Verification items for the finished model (mm, model axes). Face numbers are marked on the shaded views. A direction names the side the tool comes from. Give positions to 0.01 mm unless a question says otherwise; leave off trailing zeros. Loops run counter-clockwise (first coordinate to the right, second up) from the corner with the lowest first, then second, coordinate; pieces in that order, holes last. Notation, with made-up numbers: M -5.75,32.25 L 1.25,32.25 A21 cw 1.25,60.25 Z; hole C 29.5,6.5 d7. An arc over 180 degrees is marked long. Put each result on its own line as item: value. Start each with the question number.
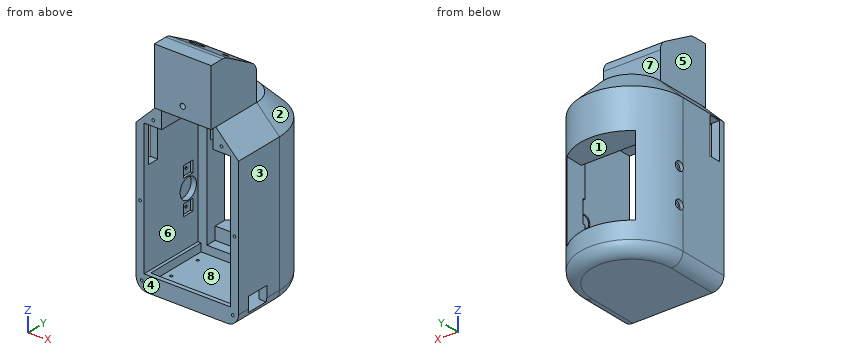
from build123d import *

# Parameters (mm, degrees)
SCHIZZO1_W                             = 90
SCHIZZO1_H                             = 150
ESTRUSIONE_ESTRUSIONE1_DEPTH           = 90
SCHIZZO4_W                             = 60
SCHIZZO4_H                             = 70
TAGLIO_ESTRUSIONE2_DEPTH               = 90
RACCORDO5_R                            = 45
RACCORDO6_R                            = 45
SMUSSO2_SIZE                           = 20
SCHIZZO7_W                             = 50
SCHIZZO7_H                             = 44.753189799
ESTRUSIONE_ESTRUSIONE2_DEPTH           = 50
SMUSSO3_SIZE                           = 20
SMUSSO3_SIZE2                          = 34.641016151
RACCORDO7_R                            = 10
RACCORDO8_R                            = 10
SCHIZZO9_W                             = 50
SCHIZZO9_H                             = 50
ESTRUSIONE_ESTRUSIONE3_DEPTH           = 5
RACCORDO9_R                            = 10
SCHIZZO13_W                            = 45
SCHIZZO13_H                            = 38.415996799
TAGLIO_ESTRUSIONE3_DEPTH               = 79.978264331
SCHIZZO14_W                            = 117.844501366
SCHIZZO14_H                            = 59.041021869
TAGLIO_ESTRUSIONE4_DEPTH               = 8
SCHIZZO18_R                            = 5
TAGLIO_ESTRUSIONE5_DEPTH               = 9
SCHIZZO16_W                            = 4
SCHIZZO16_H                            = 20
TAGLIO_ESTRUSIONE7_DEPTH               = 2
SCHIZZO23_W                            = 76
SCHIZZO23_H                            = 117.844501366
TAGLIO_ESTRUSIONE8_DEPTH               = 38
FORO_PER_VITE_M2_2_D                   = 2.4
FORO_PER_VITE_M2_2_DEPTH               = 4
FORO_PER_VITE_M4_1_D                   = 4.5
FORO_PER_VITE_M4_1_DEPTH               = 10
SCHIZZO29_W                            = 60
SCHIZZO29_H                            = 11.209863528
TAGLIO_ESTRUSIONE9_DEPTH               = 30
SCHIZZO30_W                            = 70
SCHIZZO30_H                            = 52
TAGLIO_ESTRUSIONE10_DEPTH              = 7
FORO_PER_VITE_M2_3_D                   = 2.4
FORO_PER_VITE_M2_3_DEPTH               = 4
FORO_PER_VITE_M2_3_TIP                 = 0.721032743
SCHIZZO33_W                            = 13
SCHIZZO33_H                            = 20
TAGLIO_ESTRUSIONE11_DEPTH              = 36
SCHIZZO36_W                            = 46.07976418
SCHIZZO36_H                            = 28.262497783
TAGLIO_ESTRUSIONE12_DEPTH              = 28
ESTRUSIONE_ESTRUSIONE4_REACH           = 170.388
SCHIZZO38_R                            = 6
SCHIZZO38_R_2                          = 2.5
TAGLIO_ESTRUSIONE13_DEPTH              = 28
SCHIZZO39_R                            = 9
SCHIZZO39_W                            = 10
SCHIZZO39_H                            = 10
TAGLIO_ESTRUSIONE14_DEPTH              = 2
SCHIZZO40_W                            = 32
SCHIZZO40_H                            = 10
TAGLIO_ESTRUSIONE15_DEPTH              = 10
SCHIZZO42_R                            = 4
TAGLIO_ESTRUSIONE16_DEPTH              = 3
FORO_SVASATO_PER_VITE_M2_3_D           = 2.4
FORO_SVASATO_PER_VITE_M2_3_DEPTH       = 6
FORO_SVASATO_PER_VITE_M2_3_CSINK_D     = 4.4
FORO_SVASATO_PER_VITE_M2_3_CSINK_ANGLE = 90
FORO_SVASATO_PER_VITE_M2_3_TIP         = 0.721032743
TAGLIO_ESTRUSIONE18_DEPTH              = 7
SCHIZZO53_R                            = 9
TAGLIO_ESTRUSIONE19_DEPTH              = 2.75
SCHIZZO54_W                            = 60
SCHIZZO54_H                            = 36.634637838
TAGLIO_ESTRUSIONE20_DEPTH              = 24.75


with BuildPart() as part:
    # Schizzo1 → Estrusione-Estrusione1 (new body)
    with BuildSketch(Plane(origin=(0, 0, 0), x_dir=(1, 0, 0), z_dir=(0, 1, 0))):
        Rectangle(SCHIZZO1_W, SCHIZZO1_H)
    extrude(amount=ESTRUSIONE_ESTRUSIONE1_DEPTH)

    # Schizzo4 → Taglio-Estrusione2 (cut)
    with BuildSketch(Plane(origin=(0, 90, 0), x_dir=(1, 0, 0), z_dir=(0, 1, 0))):
        with Locations((0, 15)):
            Rectangle(SCHIZZO4_W, SCHIZZO4_H)
    extrude(amount=-TAGLIO_ESTRUSIONE2_DEPTH, mode=Mode.SUBTRACT)

    # Raccordo5
    # the kernel refuses this fillet: 45 mm, written as the material it takes off along each edge
    with BuildSketch(Plane(origin=(-45, 90, -187.5), x_dir=(0, -1, 0), z_dir=(0, 0, 1))) as raccordo5_piece_1:
        with BuildLine():
            CenterArc((RACCORDO5_R, RACCORDO5_R), RACCORDO5_R, 180, 90)
            Line((0, RACCORDO5_R), (0, 0))
            Line((0, 0), (RACCORDO5_R, 0))
        make_face()
    extrude(amount=375, mode=Mode.SUBTRACT)

    # Raccordo6
    # the kernel refuses this fillet: 45 mm, written as the material it takes off along each edge
    with BuildSketch(Plane(origin=(45, 90, 187.5), x_dir=(0, -1, 0), z_dir=(0, 0, -1))) as raccordo6_piece_1:
        with BuildLine():
            CenterArc((RACCORDO6_R, RACCORDO6_R), RACCORDO6_R, 180, 90)
            Line((0, RACCORDO6_R), (0, 0))
            Line((0, 0), (RACCORDO6_R, 0))
        make_face()
    extrude(amount=375, mode=Mode.SUBTRACT)

    # Smusso2
    smusso2_edges = [part.edges().sort_by_distance(p)[0] for p in [
        (-45, 22.5, 75),
        (0, 90, 75),
        (45, 22.5, 75),
        (0, 90, 75),
    ]]
    chamfer(smusso2_edges, length=SMUSSO2_SIZE)

    # Schizzo7 → Estrusione-Estrusione2 (add)
    with BuildSketch(Plane.XY.offset(75)):
        with Locations((0, 22.3765949)):
            Rectangle(SCHIZZO7_W, SCHIZZO7_H)
    extrude(amount=ESTRUSIONE_ESTRUSIONE2_DEPTH)

    # Smusso3
    smusso3_edges = [part.edges().sort_by_distance(p)[0] for p in [
        (0, 44.753189799, 125),
    ]]
    smusso3_side = [part.faces().sort_by_distance(p)[0] for p in [
        (0, 44.753189799, 100),
    ]]
    chamfer(smusso3_edges, length=SMUSSO3_SIZE, length2=SMUSSO3_SIZE2, reference=smusso3_side[0])

    # Raccordo7
    raccordo7_edges = [part.edges().sort_by_distance(p)[0] for p in [
        (0, 44.753189799, 105),
    ]]
    fillet(raccordo7_edges, radius=RACCORDO7_R)

    # Raccordo8
    raccordo8_edges = [part.edges().sort_by_distance(p)[0] for p in [
        (0, 10.112173648, 125),
    ]]
    fillet(raccordo8_edges, radius=RACCORDO8_R)

    # Schizzo9 → Estrusione-Estrusione3 (add)
    with BuildSketch(Plane.XZ):
        with Locations((0, 100)):
            Rectangle(SCHIZZO9_W, SCHIZZO9_H)
    extrude(amount=ESTRUSIONE_ESTRUSIONE3_DEPTH)

    # Raccordo9
    raccordo9_edges = [part.edges().sort_by_distance(p)[0] for p in [
        (-45, 22.5, -75),
        (0, 90, -75),
        (45, 22.5, -75),
        (0, 90, -75),
    ]]
    fillet(raccordo9_edges, radius=RACCORDO9_R)

    # Schizzo13 → Taglio-Estrusione3 (cut)
    with BuildSketch(Plane(origin=(0, 0, 20), x_dir=(-1, 0, 0), z_dir=(0, 0, -1))):
        with Locations((0, 19.2079984)):
            Rectangle(SCHIZZO13_W, SCHIZZO13_H)
    extrude(amount=-TAGLIO_ESTRUSIONE3_DEPTH, mode=Mode.SUBTRACT)

    # Schizzo14 → Taglio-Estrusione4 (cut)
    with BuildSketch(Plane.ZY.offset(-30)):
        with Locations((-2.287612845, 29.520510935)):
            Rectangle(SCHIZZO14_W, SCHIZZO14_H)
    taglio_estrusione4 = extrude(amount=-TAGLIO_ESTRUSIONE4_DEPTH, mode=Mode.SUBTRACT)

    # Specchia1: Taglio-Estrusione4 across plane
    add(taglio_estrusione4.mirror(Plane(origin=(0, 0, 0), x_dir=(0, 0, 1), z_dir=(1, 0, 0))), mode=Mode.SUBTRACT)

    # Schizzo18 → Taglio-Estrusione5 (cut)
    with BuildSketch(Plane.ZY.offset(-30)):
        with Locations((-15, 48.541019662)):
            Circle(SCHIZZO18_R)
    extrude(amount=-TAGLIO_ESTRUSIONE5_DEPTH, mode=Mode.SUBTRACT)

    # Schizzo16 → Taglio-Estrusione7 (cut)
    with BuildSketch(Plane.XZ.offset(-59.041021869)):
        with Locations((32, -15)):
            Rectangle(SCHIZZO16_W, SCHIZZO16_H)
    extrude(amount=-TAGLIO_ESTRUSIONE7_DEPTH, mode=Mode.SUBTRACT)

    # Schizzo23 → Taglio-Estrusione8 (cut)
    with BuildSketch(Plane.XZ):
        with Locations((0, -2.287612845)):
            Rectangle(SCHIZZO23_W, SCHIZZO23_H)
    extrude(amount=-TAGLIO_ESTRUSIONE8_DEPTH, mode=Mode.SUBTRACT)

    # Foro per Vite M2-2
    with Locations(Plane(origin=(0, 0, 0), x_dir=(-1, 0, 0), z_dir=(0, -1, 0))):
        with Locations((40, 67), (30, -61.514718626), (-30, -61.514718626), (-40, 67), (-41.5, 5), (41.5, 5)):
            Hole(FORO_PER_VITE_M2_2_D / 2, depth=FORO_PER_VITE_M2_2_DEPTH)

    # Foro per Vite M4-1
    with Locations(Plane(origin=(0, -5, 84.779580177), x_dir=(0, 0, -1), z_dir=(0, -1, 0))):
        with Locations((0, 0)):
            Hole(FORO_PER_VITE_M4_1_D / 2, depth=FORO_PER_VITE_M4_1_DEPTH)

    # Schizzo29 → Taglio-Estrusione9 (cut)
    with BuildSketch(Plane.XZ.offset(-38)):
        with Locations((0, -55.604931764)):
            Rectangle(SCHIZZO29_W, SCHIZZO29_H)
    extrude(amount=-TAGLIO_ESTRUSIONE9_DEPTH, mode=Mode.SUBTRACT)

    # Schizzo30 → Taglio-Estrusione10 (cut)
    with BuildSketch(Plane.XY.offset(-61.209863528)):
        with Locations((3, 29.778767455)):
            Rectangle(SCHIZZO30_W, SCHIZZO30_H)
    extrude(amount=-TAGLIO_ESTRUSIONE10_DEPTH, mode=Mode.SUBTRACT)

    # Foro per Vite M2-3
    with Locations(Plane.XY.offset(-68.209863528)):
        with Locations((-29.5, 48.278767455), (-29.5, 19.278767455), (22.5, 6.278767455), (22.5, 53.278767455)):
            Hole(FORO_PER_VITE_M2_3_D / 2, depth=FORO_PER_VITE_M2_3_DEPTH)
            with Locations((0, 0, -(FORO_PER_VITE_M2_3_DEPTH + FORO_PER_VITE_M2_3_TIP / 2))):  # 118° drill point
                Cone(0, FORO_PER_VITE_M2_3_D / 2, FORO_PER_VITE_M2_3_TIP, mode=Mode.SUBTRACT)

    # Schizzo33 → Taglio-Estrusione11 (cut)
    with BuildSketch(Plane.ZY.offset(-38)):
        with Locations((-61.709863528, 21)):
            Rectangle(SCHIZZO33_W, SCHIZZO33_H)
    extrude(amount=-TAGLIO_ESTRUSIONE11_DEPTH, mode=Mode.SUBTRACT)

    # Schizzo36 → Taglio-Estrusione12 (cut)
    with BuildSketch(Plane(origin=(0, 56.654631148, 98.128699633), x_dir=(1, 0, 0), z_dir=(0, 0.5000000000000012, 0.8660254037844378))):
        with Locations((0, -35.289606117)):
            Rectangle(SCHIZZO36_W, SCHIZZO36_H)
    extrude(amount=-TAGLIO_ESTRUSIONE12_DEPTH, mode=Mode.SUBTRACT)

    # Schizzo37 → Estrusione-Estrusione4 (add, up to next)
    with BuildSketch(Plane.ZY.offset(-23.03988209), mode=Mode.PRIVATE) as estrusione_estrusione4_sk1:
        Polygon((122.839127138, 13.854915234), (108.707878246, 38.330956288), (106.809101084, 37.234696782), (120.940349975, 12.758655728), align=None)
    estrusione_estrusione4_tool1 = extrude(estrusione_estrusione4_sk1.sketch, amount=ESTRUSIONE_ESTRUSIONE4_REACH, mode=Mode.PRIVATE) - part.part
    add(estrusione_estrusione4_tool1.solids().sort_by_distance((23.039882, 25.544806, 114.824114))[0])

    # Schizzo38 → Taglio-Estrusione13 (cut)
    with BuildSketch(Plane(origin=(0, 56.654631148, 98.128699633), x_dir=(1, 0, 0), z_dir=(0, 0.5000000000000013, 0.8660254037844379))):
        with Locations(Location((-12.5, -35.289606117, 0), (0, 0, 270))):
            Circle(SCHIZZO38_R)
        with Locations(Location((12.5, -35.289606117, 0), (0, 0, 270))):
            Circle(SCHIZZO38_R_2)
    extrude(amount=-TAGLIO_ESTRUSIONE13_DEPTH, mode=Mode.SUBTRACT)

    # Schizzo39 → Taglio-Estrusione14 (cut)
    with BuildSketch(Plane(origin=(-38, 0, 0), x_dir=(0, 0, -1), z_dir=(1, 0, 0))):
        with Locations(Location((15, 48.541019662, 0), (0, 0, 90))):
            Circle(SCHIZZO39_R)
        with Locations((0, 48.541019662)):
            Rectangle(SCHIZZO39_W, SCHIZZO39_H)
        with Locations((30, 48.541019662)):
            Rectangle(SCHIZZO39_W, SCHIZZO39_H)
    extrude(amount=-TAGLIO_ESTRUSIONE14_DEPTH, mode=Mode.SUBTRACT)

    # Schizzo40 → Taglio-Estrusione15 (cut)
    with BuildSketch(Plane.ZY.offset(45)):
        with Locations((38, 10)):
            Rectangle(SCHIZZO40_W, SCHIZZO40_H)
    extrude(amount=-TAGLIO_ESTRUSIONE15_DEPTH, mode=Mode.SUBTRACT)

    # Schizzo42 → Taglio-Estrusione16 (cut)
    with BuildSketch(Plane.ZY.offset(45)):
        with Locations((-30, 48.541019662)):
            Circle(SCHIZZO42_R)
        with Locations((0, 48.541019662)):
            Circle(SCHIZZO42_R)
    extrude(amount=-TAGLIO_ESTRUSIONE16_DEPTH, mode=Mode.SUBTRACT)

    # Foro svasato per Vite M2-3
    with Locations(Plane.ZY.offset(42)):
        with Locations((-30, 48.541019662), (0, 48.541019662)):
            CounterSinkHole(FORO_SVASATO_PER_VITE_M2_3_D / 2, FORO_SVASATO_PER_VITE_M2_3_CSINK_D / 2, depth=FORO_SVASATO_PER_VITE_M2_3_DEPTH, counter_sink_angle=FORO_SVASATO_PER_VITE_M2_3_CSINK_ANGLE)
            with Locations((0, 0, -(FORO_SVASATO_PER_VITE_M2_3_DEPTH + FORO_SVASATO_PER_VITE_M2_3_TIP / 2))):  # 118° drill point
                Cone(0, FORO_SVASATO_PER_VITE_M2_3_D / 2, FORO_SVASATO_PER_VITE_M2_3_TIP, mode=Mode.SUBTRACT)

    # Schizzo50 → Taglio-Estrusione18 (cut)
    with BuildSketch(Plane.XY.offset(-61.209863528)):
        Polygon((38, 59.041021869), (38, 55.778767455), (-32, 55.778767455), (-32, 3.778767455), (-35.181345979, 3.778767455), (-35.181345979, 59.041021869), align=None)
    extrude(amount=-TAGLIO_ESTRUSIONE18_DEPTH, mode=Mode.SUBTRACT)

    # Schizzo53 → Taglio-Estrusione19 (cut)
    with BuildSketch(Plane(origin=(-40, 0, 0), x_dir=(0, 0, -1), z_dir=(1, 0, 0))):
        with Locations(Location((15, 48.541019662, 0), (0, 0, 90))):
            Circle(SCHIZZO53_R)
    extrude(amount=-TAGLIO_ESTRUSIONE19_DEPTH, mode=Mode.SUBTRACT)

    # Schizzo54 → Taglio-Estrusione20 (cut)
    with BuildSketch(Plane.XZ.offset(-38)):
        with Locations((0, 38.317318919)):
            Rectangle(SCHIZZO54_W, SCHIZZO54_H)
    extrude(amount=-TAGLIO_ESTRUSIONE20_DEPTH, mode=Mode.SUBTRACT)


solid = part.part
Q1. Cross-section at D-D, the plane z = 94. Record the boundary of the cut face in (x, y), then the cut area to 3 significant figures.
Q2. Cross-section at A-A, the plane z = 11. Record the boundary of the cut face in (x, y).
Q3. Release check for a two-part mould opening along Z. For the marked faces 1, 2 and 3 record: pulls with the +Z half, pulls with the -Z half, needs draft (parallel to the pull), parting line crosses it, or undercut.
Q4. Cross-section at B-B, the plane x = 0. State how many separate pieces and enclosed holes the cut face has, then the cut area to 3 significant figures.
Q5. Cross-section at C-C, the plane z = 45.5. Record the boundary of the cut face in (x, y).
Q6. Scan lines: L1, parallel to X at y = 27, z = -19; L2, parallel to Y at x = -9.5, z = 83.5; L3, parallel to Z at x = -11, y = 34. Record each from-to range of solid material in increasing order.
Q7. Set-up check for the marked faces 4, 5, 6, 7 and 8: record each of +Z, -Z, +X, -X, +Y, -Y from which the full face is reachable in a straight line by a thin tool's end or side.
Q8. Go/stop test with flat-tipped pins: pin 1 (3 mm diameter, centred on x = -27.5, z = -17.5, fed in from -Y) (1 decimal); pin 2 (2.5 mm diameter, centred on y = 48, z = -30.5, fed in from -X); pin 3 (0.9 mm diameter, centred on x = 5, z = 99.5, fed in from +Y); pin 4 (5.5 mm diameter, centred on x = -40.5, y = 9, fed in from +Z). Record where each tip stops, or that it passes through.
Ans:
1. outline: M -25,-5 L 25,-5 L 25,44.75 L -25,44.75 Z; hole M -23.04,7.81 L -22.5,7.81 L -22.5,0 L 22.5,0 L 22.5,7.81 L 23.04,7.81 L 23.04,29.84 L 22.5,29.84 L 22.5,38.42 L -22.5,38.42 L -22.5,29.84 L -23.04,29.84 Z
1. area: 735 mm^2
2. outline: M -45,0 L -38,0 L -38,59.04 L -30,59.04 L -30,78.54 A45 ccw -45,45 Z; M 30,59.04 L 38,59.04 L 38,0 L 45,0 L 45,45 A45 ccw 30,78.54 Z
3. face 1: undercut
3. face 2: pulls with the +Z half
3. face 3: needs draft
4. separate pieces: 3
4. enclosed holes: 0
4. area: 3,520 mm^2
5. outline: M -45,0 L -38,0 L -38,5 L -45,5 Z; M -45,15 L -38,15 L -38,59.04 L -30,59.04 L -30,62.75 L 30,62.75 L 30,59.04 L 38,59.04 L 38,0 L 45,0 L 45,45 A45 ccw -45,45 Z
6. L1: x = -45 to -38, 38 to 45
6. L2: y = -5 to 0, 38.42 to 44.75
6. L3: z = -75 to -68.21, 99.98 to 101.21, 108.68 to 111.21
7. face 4: -Z, +X, -X, -Y
7. face 5: +Z, -X, +Y, -Y
7. face 6: -Y
7. face 7: +Z, +X, -X, +Y
7. face 8: none
8. pin 1: passes through
8. pin 2: stops at x = -41.79
8. pin 3: stops at y = 44.75
8. pin 4: stops at z = 62.25
